```python
from build123d import *

# Parameters (mm, degrees)
SKETCH1_R           = 0.25
BOSS_EXTRUDE1_DEPTH = 0.75
SKETCH2_R           = 0.25
BOSS_EXTRUDE2_DEPTH = 4.25
SKETCH3_R           = 0.25
BOSS_EXTRUDE3_DEPTH = 4.25


with BuildPart() as part:
    # Sketch1 → Boss-Extrude1 (new body, symmetric)
    with BuildSketch(Plane(origin=(0, 0, 0), x_dir=(1, 0, 0), z_dir=(0, 1, 0))):
        Circle(SKETCH1_R)
    extrude(amount=BOSS_EXTRUDE1_DEPTH, both=True)

    # Sketch2 → Boss-Extrude2 (add)
    with BuildSketch(Plane(origin=(0, 0.75, 0), x_dir=(1, 0, 0), z_dir=(0, 1, 0))):
        Circle(SKETCH2_R)
    extrude(amount=BOSS_EXTRUDE2_DEPTH)

    # Sketch3 → Boss-Extrude3 (add)
    with BuildSketch(Plane.XZ.offset(0.75)):
        Circle(SKETCH3_R)
    extrude(amount=BOSS_EXTRUDE3_DEPTH)


solid = part.part
```
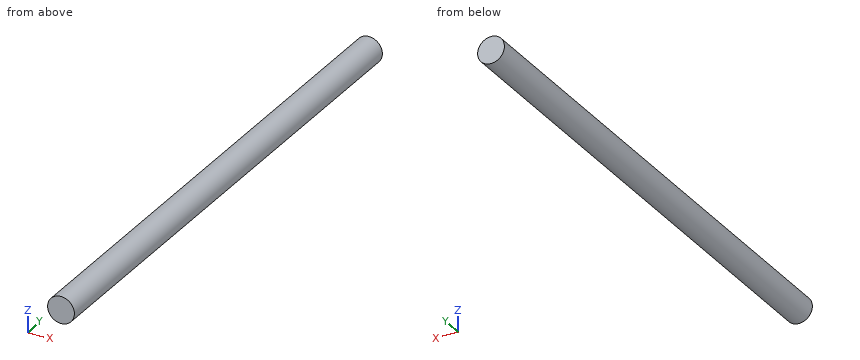
Part model, mm, in its own coordinate system. Round coordinates to 2 decimals unless told otherwise and drop trailing zeros. Loops run counter-clockwise (first coordinate to the right, second up) from the corner with the lowest first, then second, coordinate; pieces in that order, holes last.
Item 1: Cut at A-A, the plane x = 0.15. Give the cut face in (y, z).
Item 2: Cut at C-C, the plane z = -0.1. Give the cut face in (x, y), then the cut area to 3 significant figures.
Item 3: Drill centre lines: line 1 (X direction, y = -2.25, z = -0.1); line 2 (Z direction, x = -0.15, y = -3.5). Where is each one in solid material? Low to high.
Item 4: Cut at B-B, the plane y = 3.5. Give the cut face in (x, z).
A:
1. outline: (-5, -0.2) - (5, -0.2) - (5, 0.2) - (-5, 0.2) - close
2. outline: (-0.23, -5) - (0.23, -5) - (0.23, 5) - (-0.23, 5) - close
2. area: 4.58 mm2
3. line 1: x = -0.23 to 0.23
3. line 2: z = -0.2 to 0.2
4. outline: circle Ø0.5 at (0, 0)
